Geometry check sheet. Reference: the model listing, model coordinates, mm. Face numbers are marked on the shaded views. A direction names the side the tool comes from. Round coordinates to 2 decimals unless told otherwise and drop trailing zeros. Write each loop counter-clockwise with the first axis right and the second up, starting at its lowest first coordinate (ties: lowest second). Pieces come first, ordered by that corner, then holes. Notation, with made-up numbers: (-19, -20.75) -> (-14, -20.75) arc R37 ccw to (-14, 16.25) -> close; hole circle Ø6 at (43, 87). An arc over 180 degrees is marked (long way). Put each result on its own line as item: value. Start each with the question number.
from build123d import *

# Parameters (mm, degrees)
ESQUISSE1_R                         = 1.65
ESQUISSE1_R_2                       = 2.5
ESQUISSE1_W                         = 4.6
ESQUISSE1_H                         = 8.6
ESQUISSE1_R_3                       = 11.1
BOSS_EXTRU_1_DEPTH                  = 12
CHANFREIN1_SIZE                     = 2
ENL_V_MAT_EXTRU_1_REACH             = 56.08
ESQUISSE2_R                         = 2.65
ENL_V_MAT_EXTRU_1_DIRECTION_2_DEPTH = 55.07996437
R_P_TITION_CIRCULAIRE1_COUNT        = 2
ENL_V_MAT_EXTRU_3_DEPTH             = 8


with BuildPart() as part:
    # Esquisse1 → Boss.-Extru.1 (new body)
    with BuildSketch(Plane.XY):
        with BuildLine():
            Line((-23.741352507, 6.2), (-23.741352507, -6.2))
            Line((-23.741352507, -6.2), (-29.147898724, -6.2))
            ThreePointArc((-29.147898724, -6.2), (-21.071782079, -21.071782079), (-6.2, -29.147898724))
            ThreePointArc((-6.2, -29.147898724), (0, -29.8), (6.2, -29.147898724))
            ThreePointArc((6.2, -29.147898724), (21.071782079, -21.071782079), (29.147898724, -6.2))
            Line((29.147898724, -6.2), (23.741352507, -6.2))
            Line((23.741352507, -6.2), (23.741352507, 6.2))
            Line((23.741352507, 6.2), (29.147898724, 6.2))
            ThreePointArc((29.147898724, 6.2), (0, 29.8), (-29.147898724, 6.2))
            Line((-29.147898724, 6.2), (-23.741352507, 6.2))
        make_face()
        with Locations((-15.5, -15.5)):
            Circle(ESQUISSE1_R, mode=Mode.SUBTRACT)
        with Locations((-8.029746973, -17.219847954)):
            Circle(ESQUISSE1_R_2, mode=Mode.SUBTRACT)
        with Locations((-17.219847954, -8.029746973)):
            Circle(ESQUISSE1_R_2, mode=Mode.SUBTRACT)
        with Locations((0, -19)):
            Circle(ESQUISSE1_R_2, mode=Mode.SUBTRACT)
        with Locations((8.029746973, -17.219847954)):
            Circle(ESQUISSE1_R_2, mode=Mode.SUBTRACT)
        with Locations((15.5, -15.5)):
            Circle(ESQUISSE1_R, mode=Mode.SUBTRACT)
        with Locations((17.219847954, -8.029746973)):
            Circle(ESQUISSE1_R_2, mode=Mode.SUBTRACT)
        with Locations((16.656153343, -0.3)):
            Rectangle(ESQUISSE1_W, ESQUISSE1_H, mode=Mode.SUBTRACT)
        with Locations((-16.656153343, 0.3)):
            Rectangle(ESQUISSE1_W, ESQUISSE1_H, mode=Mode.SUBTRACT)
        with Locations((-17.219847954, 8.029746973)):
            Circle(ESQUISSE1_R_2, mode=Mode.SUBTRACT)
        with Locations((-15.5, 15.5)):
            Circle(ESQUISSE1_R, mode=Mode.SUBTRACT)
        with Locations((-8.029746973, 17.219847954)):
            Circle(ESQUISSE1_R_2, mode=Mode.SUBTRACT)
        Circle(ESQUISSE1_R_3, mode=Mode.SUBTRACT)
        with Locations((17.219847954, 8.029746973)):
            Circle(ESQUISSE1_R_2, mode=Mode.SUBTRACT)
        with Locations((0, 19)):
            Circle(ESQUISSE1_R_2, mode=Mode.SUBTRACT)
        with Locations((8.029746973, 17.219847954)):
            Circle(ESQUISSE1_R_2, mode=Mode.SUBTRACT)
        with Locations((15.5, 15.5)):
            Circle(ESQUISSE1_R, mode=Mode.SUBTRACT)
    extrude(amount=BOSS_EXTRU_1_DEPTH)

    # Chanfrein1
    chanfrein1_edges = [part.edges().sort_by_distance(p)[0] for p in [
        (13.85, 15.5, 12),
        (13.85, -15.5, 12),
        (-17.15, -15.5, 12),
        (-17.15, 15.5, 12),
    ]]
    chamfer(chanfrein1_edges, length=CHANFREIN1_SIZE)

    # Esquisse2 → Enlèv. mat.-Extru.1 (cut, up to next)
    with BuildSketch(Plane.ZY.offset(14.356153343), mode=Mode.PRIVATE) as enl_v_mat_extru_1_sk1:
        with Locations((7, 0)):
            Circle(ESQUISSE2_R)
    enl_v_mat_extru_1_tool1 = extrude(enl_v_mat_extru_1_sk1.sketch, amount=-ENL_V_MAT_EXTRU_1_REACH, mode=Mode.PRIVATE) & part.part
    enl_v_mat_extru_1 = enl_v_mat_extru_1_tool1.solids().sort_by_distance((-14.356153, 0, 7))[0]
    add(enl_v_mat_extru_1, mode=Mode.SUBTRACT)

    # Esquisse2 → Enlèv. mat.-Extru.1 direction 2 (cut)
    with BuildSketch(Plane.ZY.offset(14.356153343)):
        with Locations((7, 0)):
            Circle(ESQUISSE2_R)
    enl_v_mat_extru_1_direction_2 = extrude(amount=ENL_V_MAT_EXTRU_1_DIRECTION_2_DEPTH, mode=Mode.SUBTRACT)

    # Répétition circulaire1: Enlèv. mat.-Extru.1, Enlèv. mat.-Extru.1 direction 2 ×2 about axis
    r_p_tition_circulaire1_axis = Axis((0, 0, 12), (0, 0, 1))
    add([enl_v_mat_extru_1.rotate(r_p_tition_circulaire1_axis, i * 360 / R_P_TITION_CIRCULAIRE1_COUNT) for i in range(1, R_P_TITION_CIRCULAIRE1_COUNT)], mode=Mode.SUBTRACT)
    add([enl_v_mat_extru_1_direction_2.rotate(r_p_tition_circulaire1_axis, i * 360 / R_P_TITION_CIRCULAIRE1_COUNT) for i in range(1, R_P_TITION_CIRCULAIRE1_COUNT)], mode=Mode.SUBTRACT)

    # Esquisse4 → Enlèv. mat.-Extru.3 (cut)
    with BuildSketch(Plane(origin=(0, 0, 0), x_dir=(-1, 0, 0), z_dir=(0, 0, -1))):
        Polygon((0, 14.381197846), (4, 16.690598923), (4, 21.309401077), (0, 23.618802154), (-4, 21.309401077), (-4, 16.690598923), align=None)
        Polygon((0, -14.381197846), (-4, -16.690598923), (-4, -21.309401077), (0, -23.618802154), (4, -21.309401077), (4, -16.690598923), align=None)
    extrude(amount=-ENL_V_MAT_EXTRU_3_DEPTH, mode=Mode.SUBTRACT)


solid = part.part
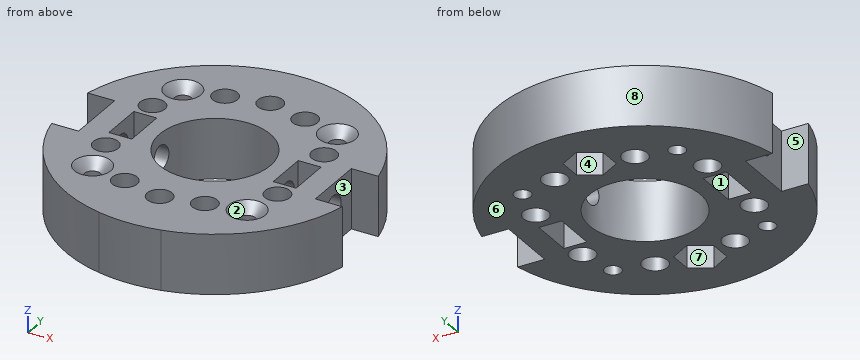
(1) Sectioned sample at A-A (z = 10.75). State how many separate pieces and enclosed holes the cut face has, and give its area (3 significant figures).
(2) Sectioned sample at C-C (x = 15.5). Record the cut outline in (y, z), and give its area (3 significant figures).
(3) Go/stop test with flat-tipped pins: pin 1 Ø2.5 at (y, z) = (0, 5.5) entering from +X; pin 2 Ø10 at (x, y) = (14.5, -14.5) entering from +Z; pin 3 Ø3.5 at (y, z) = (-18, 6) entering from +X; pin 4 Ø3 at (x, y) = (-17.22, 8.03) entering from +Z (3 decimals). Record where each tip stops, or that it passes through.
(4) Sectioned sample at D-D (y = 7). Record the cut outline in (x, z).
(5) Sectioned sample at B-B (y = 15.5). Record the cut outline in (x, z), and give its area (3 significant figures).
(6) Mould release check, pull along Y, two halves, no side actions. Record for the marked faces 6, 7 and 8: +Y half, -Y half, draft (parallel to the pull), parting line (faces both ways), or undercut.
(7) Set-up check for the marked faces 1, 2, 3, 4 and 5: record each of +Z, -Z, +X, -X, +Y, -Y from which the full face is reachable in a straight line by a thin tool's end or side.
(8) Material ranges on L1, parallel to Y at x = 0, z = 2.75; L2, parallel to X at y = -18, z = 3; L3, parallel to Y at x = 3.5, z = 5, recorded low to high. Write a range as from..to.
Found:
1. separate pieces: 1
1. enclosed holes: 17
1. area: 1,910 mm2
2. outline: (-25.45, 0) -> (-17.15, 0) -> (-17.15, 10) -> (-19.15, 12) -> (-25.45, 12) -> close; (-13.85, 0) -> (-9.84, 0) -> (-9.84, 12) -> (-11.85, 12) -> (-13.85, 10) -> close; (-6.22, 0) -> (-4.6, 0) -> (-4.6, 12) -> (-6.22, 12) -> close; (4, 0) -> (6.22, 0) -> (6.22, 12) -> (4, 12) -> close; (9.84, 0) -> (13.85, 0) -> (13.85, 10) -> (11.85, 12) -> (9.84, 12) -> close; (17.15, 0) -> (25.45, 0) -> (25.45, 12) -> (19.15, 12) -> (17.15, 10) -> close
2. area: 333 mm2
3. pin 1: x = 23.74
3. pin 2: z = 12
3. pin 3: x = 24.98
3. pin 4: through
4. outline: (-28.97, 0) -> (-19.5, 0) -> (-19.5, 12) -> (-28.97, 12) -> close; (-14.94, 0) -> (-8.61, 0) -> (-8.61, 12) -> (-14.94, 12) -> close; (8.61, 0) -> (14.94, 0) -> (14.94, 12) -> (8.61, 12) -> close; (19.5, 0) -> (28.97, 0) -> (28.97, 12) -> (19.5, 12) -> close
5. outline: (-25.45, 0) -> (-17.15, 0) -> (-17.15, 10) -> (-19.15, 12) -> (-25.45, 12) -> close; (-13.85, 0) -> (-9.84, 0) -> (-9.84, 12) -> (-11.85, 12) -> (-13.85, 10) -> close; (-6.22, 0) -> (-1.94, 0) -> (-1.94, 8) -> (1.94, 8) -> (1.94, 0) -> (6.22, 0) -> (6.22, 12) -> (-6.22, 12) -> close; (9.84, 0) -> (13.85, 0) -> (13.85, 10) -> (11.85, 12) -> (9.84, 12) -> close; (17.15, 0) -> (25.45, 0) -> (25.45, 12) -> (19.15, 12) -> (17.15, 10) -> close
5. area: 406 mm2
6. face 6: draft
6. face 7: undercut
6. face 8: +Y half
7. face 1: +Z, -Z
7. face 2: +Z
7. face 3: +Z, -Z, +X
7. face 4: -Z
7. face 5: +Z, -Z, -X
8. L1: -29.8..-23.62, -14.38..-11.1, 11.1..14.38, 23.62..29.8
8. L2: -23.75..-10.4, -5.65..-4, 4..5.65, 10.4..23.75
8. L3: -29.59..-21.6, -16.4..-10.53, 10.53..16.4, 21.6..29.59
